from build123d import *

# Parameters (mm, degrees)
BOSS_EXTRUDE1_DEPTH = 3.175
SKETCH3_W           = 3.175
SKETCH3_H           = 11.825
SKETCH3_W_2         = 11.35
SKETCH3_H_2         = 3.175
SKETCH3_W_3         = 25
SKETCH3_H_3         = 49.488701784
SKETCH3_H_4         = 10
SKETCH3_W_4         = 10
CUT_EXTRUDE2_DEPTH  = 4.1750001
FILLET1_R           = 2.5


with BuildPart() as part:
    # Sketch1 → Boss-Extrude1 (new body)
    with BuildSketch(Plane(origin=(0, 0, 0), x_dir=(1, 0, 0), z_dir=(0, 1, 0))):
        with BuildLine():
            add(Edge.make_bspline(
                [(0, 0), (0, 36), (20.385499073, 62.552567554), (40.487505944, 65), (42.5, 65)],
                knots=[0, 0, 0, 0, 0.452811163, 0.503123514, 0.503123514, 0.503123514, 0.503123514], degree=3))
            Line((0, 0), (42.5, 0))
            Line((42.5, 0), (42.5, 65))
        make_face()
        with BuildLine():
            Line((42.5, 65), (42.5, 0))
            Line((42.5, 0), (85, 0))
            add(Edge.make_bspline(
                [(42.5, 65), (44.487505944, 65), (64.384933097, 62.612967274), (85, 36), (85, 0)],
                knots=[0.503123514, 0.503123514, 0.503123514, 0.503123514, 0.552811163, 1, 1, 1, 1], degree=3))
        make_face()
    extrude(amount=BOSS_EXTRUDE1_DEPTH)

    # Sketch3 → Cut-Extrude2 (cut, through all)
    with BuildSketch(Plane(origin=(0, 3.175, 0), x_dir=(1, 0, 0), z_dir=(0, 1, 0))):
        with Locations((23.4125, 5.9125)):
            Rectangle(SKETCH3_W, SKETCH3_H)
        with Locations((61.5875, 5.9125)):
            Rectangle(SKETCH3_W, SKETCH3_H)
        with Locations((42.5, 13.4125)):
            Rectangle(SKETCH3_W_2, SKETCH3_H_2)
        with Locations((42.5, 44.744350892)):
            Rectangle(SKETCH3_W_3, SKETCH3_H_3)
        with Locations((23.4125, 50)):
            Rectangle(SKETCH3_W, SKETCH3_H_4)
        with Locations((61.5875, 50)):
            Rectangle(SKETCH3_W, SKETCH3_H_4)
        with Locations((10, 1.5875)):
            Rectangle(SKETCH3_W_4, SKETCH3_H_2)
        with Locations((75, 1.5875)):
            Rectangle(SKETCH3_W_4, SKETCH3_H_2)
    extrude(amount=-CUT_EXTRUDE2_DEPTH, mode=Mode.SUBTRACT)

    # Fillet1
    fillet1_edges = [part.edges().sort_by_distance(p)[0] for p in [
        (30, 1.5875, -61.882691036),
        (55, 1.5875, -61.855383827),
    ]]
    fillet(fillet1_edges, radius=FILLET1_R)


solid = part.part
Build history of the part. All positions in model axes, mm. A direction names the side the tool comes from. Give positions to 0.01 mm unless a question says otherwise; leave off trailing zeros. Order: outer loops, then holes, each group sorted by start corner. A loop starts at its lowest first (then second) coordinate and runs counter-clockwise, first axis right, second up. Notation, with made-up numbers: M 48,-4 L 62,-4 A24 ccw 62,15 Z; hole C 9,0.25 d4. An arc over 180 degrees is marked long. Use one line per item in the form item = value.
Q1. Slice it at A-A, the plane x = 38.5. Write the cut outline in (y, z) (3 decimals).
Conclusion:
outline = M 0,-20 L 3.175,-20 L 3.175,-15 L 0,-15 Z; M 0,-11.825 L 3.175,-11.825 L 3.175,0 L 0,0 Z
Q2. Which spindle directions (+Z, -Z, +X, -X, +Y, -Y) get a long thin tool onto all of the face, cutting with end or side? Do faces 1 (the flat face through (62, 2, -11.825)), 2 (the flat face through (60, 2, -50)), 3 (the flat face through (30, 2, -39)). Say none if no direction does.
Conclusion:
face_1 = +Z, +Y, -Y
face_2 = +Y, -Y
face_3 = -Z, +Y, -Y
Q3. Pull direction X, two halves, no side cores. Call faces 4 (the flat face through (42, 2, -11.825)), 5 (the flat face through (67, 2, 0)): released by +X, released by -X, zero draft, split by the parting line, or undercut.
Conclusion:
face_4 = undercut
face_5 = zero draft
Q4. Slice it at B-B, the plane y = 1.1. State how many separate pieces and enclosed holes the cut face has, and give its area (3 significant figures).
Conclusion:
separate_pieces = 1
enclosed_holes = 3
area = 2,970 mm2
Q5. Pin check, flat tips, straight feed: P1, Ø1, axis at x = 12, y = 1, coming from the +Z side (3 decimals); P2, Ø1, axis at y = 2, z = -1, coming from the -X side; P3, Ø1, axis at y = 2.5, z = -19, coming from the +X side. Stop position of each tip, or through.
Conclusion:
P1 = -3.175
P2 = 0
P3 = 83.25
Q6. Wall check: probe 1 along Z at (x, y) = (40, 0.5) (3 decimals); probe 2 along X at (y, z) = (1.05, -6) (3 decimals); probe 3 along X at (y, z) = (2.85, -50.5) (3 decimals). Give the ranges that are in metal, low to high.
Conclusion:
probe_1 = -20 to -15, -11.825 to 0
probe_2 = 0.173 to 21.825, 25 to 60, 63.175 to 84.825
probe_3 = 16.11 to 21.825, 25 to 30, 55 to 60, 63.175 to 68.808
